from build123d import *

# Parameters (mm, degrees)
SKETCH1_R           = 33.8
SKETCH1_R_2         = 2.54
SKETCH1_R_3         = 2.05
SKETCH1_R_4         = 0.75
SKETCH1_W           = 3.048
SKETCH1_H           = 19.05
SKETCH1_W_2         = 19.05
SKETCH1_H_2         = 3.048
BOSS_EXTRUDE1_DEPTH = 6.35
BOSS_EXTRUDE2_DEPTH = 6.35
FILLET1_R           = 2.54


with BuildPart() as part:
    # Sketch1 → Boss-Extrude1 (new body)
    with BuildSketch(Plane.XY):
        Circle(SKETCH1_R)
        with Locations((14.36, 24.872249597)):
            Circle(SKETCH1_R_2, mode=Mode.SUBTRACT)
        with Locations((20.308106756, 20.308106756)):
            Circle(SKETCH1_R_2, mode=Mode.SUBTRACT)
        with Locations((24.872249597, 14.36)):
            Circle(SKETCH1_R_2, mode=Mode.SUBTRACT)
        with Locations((27.741389731, 7.433282975)):
            Circle(SKETCH1_R_2, mode=Mode.SUBTRACT)
        with Locations((28.72, 0)):
            Circle(SKETCH1_R_2, mode=Mode.SUBTRACT)
        with Locations((27.741389731, -7.433282975)):
            Circle(SKETCH1_R_2, mode=Mode.SUBTRACT)
        with Locations((24.872249597, -14.36)):
            Circle(SKETCH1_R_2, mode=Mode.SUBTRACT)
        with Locations((20.308106756, -20.308106756)):
            Circle(SKETCH1_R_2, mode=Mode.SUBTRACT)
        with Locations((14.36, -24.872249597)):
            Circle(SKETCH1_R_2, mode=Mode.SUBTRACT)
        with Locations((7.433282975, -27.741389731)):
            Circle(SKETCH1_R_2, mode=Mode.SUBTRACT)
        with Locations((0, -28.72)):
            Circle(SKETCH1_R_2, mode=Mode.SUBTRACT)
        with Locations((-7.433282975, -27.741389731)):
            Circle(SKETCH1_R_2, mode=Mode.SUBTRACT)
        with Locations((-14.36, -24.872249597)):
            Circle(SKETCH1_R_2, mode=Mode.SUBTRACT)
        with Locations((-20.308106756, -20.308106756)):
            Circle(SKETCH1_R_2, mode=Mode.SUBTRACT)
        with Locations((-24.872249597, -14.36)):
            Circle(SKETCH1_R_2, mode=Mode.SUBTRACT)
        with Locations((-27.741389731, -7.433282975)):
            Circle(SKETCH1_R_2, mode=Mode.SUBTRACT)
        with Locations((-28.72, 0)):
            Circle(SKETCH1_R_2, mode=Mode.SUBTRACT)
        with Locations((-27.741389731, 7.433282975)):
            Circle(SKETCH1_R_2, mode=Mode.SUBTRACT)
        with Locations((-24.872249597, 14.36)):
            Circle(SKETCH1_R_2, mode=Mode.SUBTRACT)
        with Locations((-20.308106756, 20.308106756)):
            Circle(SKETCH1_R_2, mode=Mode.SUBTRACT)
        with Locations((-14.36, 24.872249597)):
            Circle(SKETCH1_R_2, mode=Mode.SUBTRACT)
        with Locations((-7.433282975, 27.741389731)):
            Circle(SKETCH1_R_2, mode=Mode.SUBTRACT)
        with Locations((0, 28.72)):
            Circle(SKETCH1_R_2, mode=Mode.SUBTRACT)
        with Locations((7.433282975, 27.741389731)):
            Circle(SKETCH1_R_2, mode=Mode.SUBTRACT)
        Circle(SKETCH1_R_3, mode=Mode.SUBTRACT)
        with Locations((11.561195872, 11.561195872)):
            Circle(SKETCH1_R_4, mode=Mode.SUBTRACT)
        with Locations((9.439875529, 9.439875529)):
            Circle(SKETCH1_R_4, mode=Mode.SUBTRACT)
        with Locations((7.318555185, 7.318555185)):
            Circle(SKETCH1_R_4, mode=Mode.SUBTRACT)
        with Locations((5.197234842, 5.197234842)):
            Circle(SKETCH1_R_4, mode=Mode.SUBTRACT)
        with Locations((11.561195872, -11.561195872)):
            Circle(SKETCH1_R_4, mode=Mode.SUBTRACT)
        with Locations((9.439875529, -9.439875529)):
            Circle(SKETCH1_R_4, mode=Mode.SUBTRACT)
        with Locations((7.318555185, -7.318555185)):
            Circle(SKETCH1_R_4, mode=Mode.SUBTRACT)
        with Locations((5.197234842, -5.197234842)):
            Circle(SKETCH1_R_4, mode=Mode.SUBTRACT)
        with Locations((-11.561195872, -11.561195872)):
            Circle(SKETCH1_R_4, mode=Mode.SUBTRACT)
        with Locations((-9.439875529, -9.439875529)):
            Circle(SKETCH1_R_4, mode=Mode.SUBTRACT)
        with Locations((-7.318555185, -7.318555185)):
            Circle(SKETCH1_R_4, mode=Mode.SUBTRACT)
        with Locations((-5.197234842, -5.197234842)):
            Circle(SKETCH1_R_4, mode=Mode.SUBTRACT)
        with Locations((-11.561195872, 11.561195872)):
            Circle(SKETCH1_R_4, mode=Mode.SUBTRACT)
        with Locations((-9.439875529, 9.439875529)):
            Circle(SKETCH1_R_4, mode=Mode.SUBTRACT)
        with Locations((-7.318555185, 7.318555185)):
            Circle(SKETCH1_R_4, mode=Mode.SUBTRACT)
        with Locations((-5.197234842, 5.197234842)):
            Circle(SKETCH1_R_4, mode=Mode.SUBTRACT)
        with Locations((0, 14.115)):
            Rectangle(SKETCH1_W, SKETCH1_H, mode=Mode.SUBTRACT)
        with Locations((14.115, 0)):
            Rectangle(SKETCH1_W_2, SKETCH1_H_2, mode=Mode.SUBTRACT)
        with Locations((0, -14.115)):
            Rectangle(SKETCH1_W, SKETCH1_H, mode=Mode.SUBTRACT)
        with Locations((-14.115, 0)):
            Rectangle(SKETCH1_W_2, SKETCH1_H_2, mode=Mode.SUBTRACT)
    extrude(amount=BOSS_EXTRUDE1_DEPTH)

    # Sketch3 → Boss-Extrude2 (add)
    with BuildSketch(Plane.XY):
        with BuildLine():
            Line((-2.694076836, 37.764076836), (-7.50097995, 32.957173723))
            ThreePointArc((-7.50097995, 32.957173723), (0, 33.8), (7.50097995, 32.957173723))
            Line((7.50097995, 32.957173723), (2.694076836, 37.764076836))
            ThreePointArc((2.694076836, 37.764076836), (0, 38.88), (-2.694076836, 37.764076836))
        make_face()
    extrude(amount=BOSS_EXTRUDE2_DEPTH)

    # Fillet1
    fillet1_edges = [part.edges().sort_by_distance(p)[0] for p in [
        (-7.50097995, 32.957173723, 3.175),
        (7.50097995, 32.957173723, 3.175),
    ]]
    fillet(fillet1_edges, radius=FILLET1_R)


solid = part.part
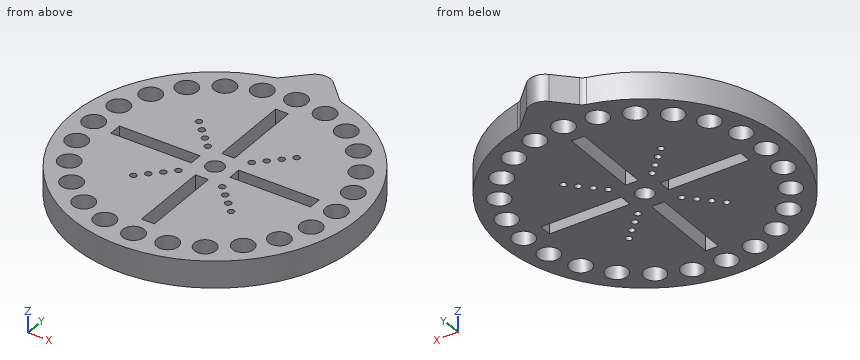
Read the model definition and answer for the solid it produces. Units are mm, in the model's axes. Give positions to 0.01 mm unless a question says otherwise; leave off trailing zeros. Loops run counter-clockwise (first coordinate to the right, second up) from the corner with the lowest first, then second, coordinate; pieces in that order, holes last. Notation, with made-up numbers: (-17.5, 54.5) -> (40.5, 54.5) arc R23 ccw to (40.5, 81.5) -> close; hole circle Ø4 at (39.5, 21.25). An arc over 180 degrees is marked (long way). Use a Markdown table: item, result.
Q1. Section B-B, the plane y = -28.72 is taken. Determine the outline of the cut face in (x, z), then the cut area to 3 significant figures.
Solved:
| item | result |
|---|---|
| outline | (-17.82, 0) -> (-9.78, 0) -> (-9.78, 6.35) -> (-17.82, 6.35) -> close; (-5.09, 0) -> (-2.54, 0) -> (-2.54, 6.35) -> (-5.09, 6.35) -> close; (2.54, 0) -> (5.09, 0) -> (5.09, 6.35) -> (2.54, 6.35) -> close; (9.78, 0) -> (17.82, 0) -> (17.82, 6.35) -> (9.78, 6.35) -> close |
| area | 135 mm^2 |
Q2. Find the intervals of material crossed by line 1 along X through (y, z) = (24, 1); line 2 along Y through (x, z) = (-28.72, 4.5); line 3 along X through (y, z) = (-18.5, 5), in increasing order.
Solved:
| item | result |
|---|---|
| line 1 | x = -23.8 to -16.75, -11.97 to 11.97, 16.75 to 23.8 |
| line 2 | y = -17.82 to -9.78, -5.09 to -2.54, 2.54 to 5.09, 9.78 to 17.82 |
| line 3 | x = -28.29 to -22.09, -18.52 to -1.52, 1.52 to 18.52, 22.09 to 28.29 |
Q3. Section D-D, the plane z = 1.5 is taken. Count the separate pieces of the cut face and the enclosed holes in it, then the cut area to 3 significant figures.
Solved:
| item | result |
|---|---|
| separate pieces | 1 |
| enclosed holes | 45 |
| area | 2,870 mm^2 |
Q4. Each of these flat-tipped pins is pushed along its axis until it touches: pin 1 (1.5 mm diameter, centred on y = -9, z = 1, fed in from -X); pin 2 (1.5 mm diameter, centred on y = -0.5, z = 3, fed in from +X); pin 3 (3 mm diameter, centred on x = -12, z = 2.5, fed in from +Y). Where does it stop, or does it pass through?
Solved:
| item | result |
|---|---|
| pin 1 | stops at x = -32.78 |
| pin 2 | stops at x = 33.8 |
| pin 3 | stops at y = 32.13 |
Q5. Section A-A, the plane x = 0 is taken. Determine the outline of the cut face in (y, z), then the cut area to 3 significant figures.
Solved:
| item | result |
|---|---|
| outline | (-33.8, 0) -> (-31.26, 0) -> (-31.26, 6.35) -> (-33.8, 6.35) -> close; (-26.18, 0) -> (-23.64, 0) -> (-23.64, 6.35) -> (-26.18, 6.35) -> close; (-4.59, 0) -> (-2.05, 0) -> (-2.05, 6.35) -> (-4.59, 6.35) -> close; (2.05, 0) -> (4.59, 0) -> (4.59, 6.35) -> (2.05, 6.35) -> close; (23.64, 0) -> (26.18, 0) -> (26.18, 6.35) -> (23.64, 6.35) -> close; (31.26, 0) -> (38.88, 0) -> (38.88, 6.35) -> (31.26, 6.35) -> close |
| area | 129 mm^2 |
Q6. Section C-C, the plane x = -14.36 is taken. Determine the outline of the cut face in (y, z).
Solved:
| item | result |
|---|---|
| outline | (-30.6, 0) -> (-27.41, 0) -> (-27.41, 6.35) -> (-30.6, 6.35) -> close; (-22.33, 0) -> (-1.52, 0) -> (-1.52, 6.35) -> (-22.33, 6.35) -> close; (1.52, 0) -> (22.33, 0) -> (22.33, 6.35) -> (1.52, 6.35) -> close; (27.41, 0) -> (30.6, 0) -> (30.6, 6.35) -> (27.41, 6.35) -> close |
